Work out the finished part from the listing and answer in its coordinate system (mm). Face numbers are marked on the shaded views. A direction names the side the tool comes from. Round coordinates to 2 decimals unless told otherwise and drop trailing zeros. Write each loop counter-clockwise with the first axis right and the second up, starting at its lowest first coordinate (ties: lowest second). Pieces come first, ordered by that corner, then holes.
1. Determine the mould class of the marked faces 1, 2 and 3 for opening direction Y: pulls with the +Y half, pulls with the -Y half, needs draft (parallel to the pull), parting line crosses it, or undercut.
2. A tool of negligible diameter and unlimited length cuts with its end or side. For the marked faces 4, 5 and 6, from which of +Z, -Z, +X, -X, +Y, -Y can it reach the whole face along a straight path? Write none if from no direction.
3. Find section B-B (z = -12.5). Count the separate pieces of the cut face and the enclosed holes in it, and give its area (3 significant figures).
4. Find section D-D (z = 2). Write down the section's boundary in (x, y).
5. Straight lines are drawn through the part: probe 1 along Y at (x, z) = (-5.5, 0.75); probe 2 along Y at (x, z) = (-5.5, 0.65); probe 3 along Z at (x, y) = (-10, 1.75). For each, find the intervals that lie inside material, in ascending order.
6. Find section C-C (y = 2). Write down the section's boundary in (x, z), and give its area (3 significant figures).
7. Find section A-A (y = 5.4). Write down the section's boundary in (x, z).
8. Flat-ended cylindrical pins translate along their axes: pin 1 Ø1.6 at (x, y) = (-6.5, 4.5) entering from -Z; pin 2 Ø10 at (x, z) = (12, -8) entering from -Y; pin 3 Ø2 at (x, z) = (-2.5, 0) entering from +Y. Find the tip coordinate at first contact, or state that the pin passes through.
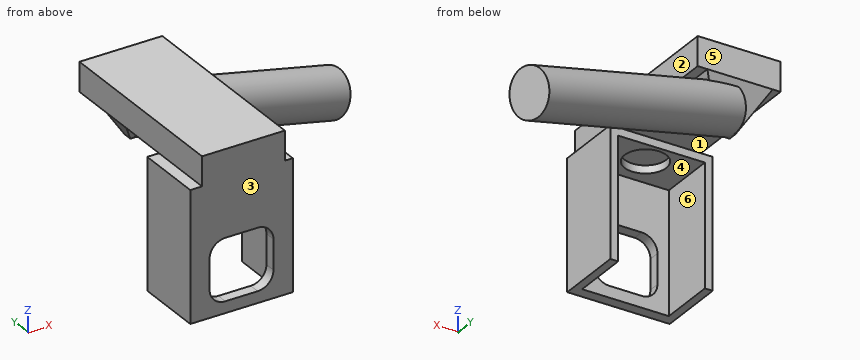
Autodesk Inventor part; units mm, degrees
ref_plane "YZ Plane" through (0, 0, 0) normal (1, 0, 0) x (0, 1, 0)
ref_plane "XZ Plane" through (0, 0, 0) normal (0, 1, 0) x (-1, 0, 0)
ref_plane "XY Plane" through (0, 0, 0) normal (0, 0, 1) x (1, 0, 0)
sketch "Sketch3" plane through (0, 0, 0) normal (0, 1, 0) x (-1, 0, 0)
  line L0 (0, 0) -> (11, 0)
  line L1 (11, 0) -> (11, -56)
  line L2 (11, -56) -> (0, -56)
  line L3 (0, -56) -> (0, 0)
  line L4 (12, 1) -> (-1, 1)
  line L5 (-1, 1) -> (-1, -57)
  line L6 (-1, -57) -> (12, -57)
  line L7 (12, -57) -> (12, 1)
  line L8 (7.55, -6.2) -> (3.45, -6.2)
  line L9 (1.45, -8.2) -> (1.45, -12)
  line L10 (3.45, -14) -> (7.55, -14)
  line L11 (9.55, -12) -> (9.55, -8.2)
  arc A0 (9.55, -8.2) -> (7.55, -6.2) centre (7.55, -8.2) ccw
  arc A1 (7.55, -14) -> (9.55, -12) centre (7.55, -12) ccw
  arc A2 (1.45, -12) -> (3.45, -14) centre (3.45, -12) ccw
  arc A3 (3.45, -6.2) -> (1.45, -8.2) centre (3.45, -8.2) ccw
  circle A4 centre (5.5, -51) radius 1
  point P0 (1.45, -14)
  point P1 (1.45, -6.2)
  point P2 (9.55, -14)
  dimension "d2" = 11
  dimension "d3" = 56
  dimension "d4" = 1
  dimension "d5" = 1
  dimension "d6" = 1
  dimension "d7" = 1
  dimension "d8" = 8.1
  dimension "d9" = 7.8
  dimension "d10" = 14
  dimension "d11" = 9.55
  dimension "d12" = 2
  dimension "d30" = 2
  dimension "d31" = 5
  dimension "d32" = 5.5
extrude "Extrusion1" add sketch "Sketch3" along normal blind 1.4 contours L0 L1 L2 L3
extrude "Extrusion3" add sketch "Sketch3" along normal blind 8.6 contours L7 L6 L5 L4
sketch "Sketch4" plane through (-12, 0, 1) normal (0, 0, 1) x (1, 0, 0)
  circle A0 centre (6.5, 5.4) radius 2.65
  line L0 (0, 0) -> (0, 8.6)
  line L1 (0, 0) -> (13, 0)
  point P0 (12, 0)
  dimension "d19" = 6.5
  dimension "d20" = 5.3
  dimension "d21" = 5.4
extrude "Extrusion4" cut sketch "Sketch4" against normal blind 8.6
sketch "Sketch5" plane through (1, 0, -57) normal (0, 0, -1) x (-1, 0, 0)
  line L0 (2.675, 6.25) -> (10.325, 6.25)
  line L1 (10.325, 6.25) -> (10.325, 3.55)
  line L2 (10.325, 3.55) -> (2.675, 3.55)
  line L3 (2.675, 3.55) -> (2.675, 6.25)
  line L4 (0, 0) -> (13, 0)
  line L5 (13, 0) -> (13, 8.6)
  point P0 (1, 0)
  dimension "d24" = 7.65
  dimension "d25" = 2.7
  dimension "d26" = 3.55
  dimension "d27" = 2.675
extrude "Extrusion5" cut sketch "Sketch5" against normal blind 8.6
sketch "Sketch6" plane through (0, 0, 0) normal (0, 1, 0) x (-1, 0, 0)
  line L0 (46.885, 6) -> (-33.7151, 6)
  line L1 (12, 1) -> (-1, 1)
  point P0 (0, 0)
  dimension "d33" = 5
ref_plane "Work Plane1" through (-46.885, 0, 6) normal (0, -0.8660254, -0.5) x (1, 0, 0)
ref_plane "Work Plane2" through (-46.885, 12.9904, 13.5) normal (0, -0.8660254, -0.5) x (1, 0, 0)
sketch "Sketch8" plane through (-46.885, 12.9904, 13.5) normal (0, -0.8660254, -0.5) x (1, 0, 0)
  line L0 (41.385, -17.0022) -> (69.5758, -27.2628)
  line L1 (47.885, -8.6301) -> (47.885, -58.8596)
  line L2 (34.885, -4.3301) -> (47.885, -4.3301)
  line L3 (46.885, -57.9936) -> (46.885, -9.4962)
  line L4 (69.5758, -27.2628) -> (70.6018, -24.4437)
  line L5 (70.6018, -24.4437) -> (42.4111, -14.1831)
  line L6 (42.4111, -14.1831) -> (41.385, -17.0022)
  point P0 (46.885, -5.1962)
  dimension "d42" = 70
  dimension "d44" = 5.5
  dimension "d45" = 30
  dimension "d46" = 3
revolve "Revolution1" add sketch "Sketch8" angle 360 about axis through (-5.5, 21.4915, -1.2243) along (0.9396926, 0.1710101, -0.2961981)
sketch "Sketch9" plane through (0, 0, 0) normal (0, 1, 0) x (-1, 0, 0)
  line L0 (12, 1) -> (-1, 1)
  line L1 (0, 1) -> (10.5086, 1)
  line L2 (10.5086, 1) -> (10.5086, 4.698)
  line L3 (10.5086, 4.698) -> (0, 4.698)
  line L4 (0, 4.698) -> (0, 1)
  point P0 (0, 0)
extrude "Extrusion6" add sketch "Sketch9" along normal blind 24.5
sketch "Sketch10" plane through (0, 8.6, 1) normal (0, 0, -1) x (-1, 0, 0)
  line L0 (0, 15.9) -> (10.5086, 15.9)
  line L1 (9.5196, 15.9) -> (1.2363, 15.9)
  line L2 (1.2363, 15.9) -> (1.2363, 8.9556)
  line L3 (1.2363, 8.9556) -> (9.5196, 8.9556)
  line L4 (9.5196, 8.9556) -> (9.5196, 15.9)
  point P0 (0, -8.6)
extrude "Extrusion7" add sketch "Sketch10" along normal blind 5 draft -30
sketch "Sketch11" plane through (0, 0, 0) normal (1, 0, 0) x (0, 1, 0)
  line L0 (17.1847, -15.4539) -> (-9.2723, -15.4539)
  line L1 (-9.2723, -15.4539) -> (-9.2723, -62.4336)
  line L2 (-9.2723, -62.4336) -> (17.1847, -62.4336)
  line L3 (17.1847, -62.4336) -> (17.1847, -15.4539)
  point P0 (0, 0)
extrude "Extrusion8" cut sketch "Sketch11" along normal through all both and the other way through all
equation "\"d11\" = 0.5 * d2 + 0.5 * d8"
equation "\"d32\" = 0.5 * d2"
equation "\"d19\" = 0.5 * d2 + d4"
equation "\"d44\" = 0.5 * d2"
properties part number "QC25BTFication_2"
Worked answers:
1. face 1: undercut
1. face 2: needs draft
1. face 3: pulls with the -Y half
2. face 4: -Z
2. face 5: +Z, +X, -X, +Y
2. face 6: -Z, +Y
3. separate pieces: 3
3. enclosed holes: 0
3. area: 25.2 mm2
4. outline: (-10.51, 0) - (0, 0) - (0, 24.5) - (-10.51, 24.5) - close
5. probe 1: y = 0 to 2.75, 8.05 to 8.6, 17.7 to 24.36
5. probe 2: y = 0 to 2.75, 8.05 to 8.6, 17.76 to 24.3
5. probe 3: z = 0 to 4.7
6. outline: (-12, -15.45) - (-11, -15.45) - (-11, 0) - (0, 0) - (0, -15.45) - (1, -15.45) - (1, 1) - (0, 1) - (0, 4.7) - (-10.51, 4.7) - (-10.51, 1) - (-12, 1) - close
6. area: 82.8 mm2
7. outline: (-12, -15.45) - (-11, -15.45) - (-11, 0) - (-8.15, 0) - (-8.15, 1) - (-2.85, 1) - (-2.85, 0) - (0, 0) - (0, -15.45) - (1, -15.45) - (1, 1) - (0, 1) - (0, 4.7) - (-10.51, 4.7) - (-10.51, 1) - (-12, 1) - close
8. pin 1: stops at z = 1
8. pin 2: stops at y = 20.85
8. pin 3: stops at y = 24.8
